Here's how the part is built. I have some questions about the finished solid (model axes, mm). A direction names the side the tool comes from. Give positions to 0.01 mm unless a question says otherwise; leave off trailing zeros. Loops run counter-clockwise (first coordinate to the right, second up) from the corner with the lowest first, then second, coordinate; pieces in that order, holes last.
Q1. I'm going to push flat-ended pins straight in: P1, Ø1.5, axis at x = -3.048, z = 0, coming from the -Y side; P2, Ø3, axis at x = -6, y = -15, coming from the -Z side; P3, Ø10, axis at x = 8, y = -18, coming from the +Z side. Where does each tip first touch, or does it pass through?
Q2. Thinking about a two-plate mould opening in Z: for faces 3 (the face through (3.25, -2.13, -0.06)), 4 (the face through (-1, -20.955, -10)), 5 (the face through (-1.83, -0.77, -0.05)), 6 (the face through (-10.418, -10.624, -3.281)), which applies, pulls with the +Z half, pulls with the -Z half, needs draft (parallel to the pull), parting line crosses it, or undercut?
Q3. Suppose I cut it at B-B (z = -3.5). List the corners of the cut face in (x, y) for me (3 decimals).
Q4. Suppose I cut it at C-C (y = -7). List the corners of the cut face in (x, z) for me, and give its area (3 significant figures).
Q5. For faces 1 (the face through (0, 0, 0)), 2 (the face through (1.885, -0.773, -0.366)), which set-ups out of +Z, -Z, +X, -X, +Y, -Y let a thin tool reach every point of the face, with its end or its side?
Q6. I need wall thicknesses on probe 1 along Y at (x, z) = (-3, 9.75) (3 decimals); probe 2 along Z at (x, y) = (0.25, -3.5); probe 3 along Z at (x, y) = (2, -8.5). Which ranges of each line are inside material? Lowest first, please.
Q7. Suppose I cut it at D-D (y = -23). List the corners of the cut face in (x, z) for me.
Q8. Suppose I cut it at A-A (x = 0). List the corners of the cut face in (y, z) for me (3 decimals), and give its area (3 significant figures).
```python
from build123d import *

# Parameters (mm, degrees)
F_2_CLEARANCE_HOLE1_D     = 2.4384
F_2_CLEARANCE_HOLE1_DEPTH = 1.524
F_2_CLEARANCE_HOLE1_TIP   = 0.732569267


with BuildPart() as part:
    # Sketch1 → Revolve1 (revolve)
    with BuildSketch(Plane.XY):
        with BuildLine():
            Line((0, 0), (-10.922, 0))
            Line((-10.922, 0), (-10.922, -20.955))
            Line((-10.922, -20.955), (-9.525, -20.955))
            ThreePointArc((-9.525, -20.955), (-6.735192091, -27.690192091), (0, -30.48))
            Line((0, -30.48), (0, 0))
        make_face()
    revolve(axis=Axis((0, 0, 0), (0, -1, 0)))

    # #2 Clearance Hole1
    with Locations(Plane(origin=(0, 0, 0), x_dir=(1, 0, 0), z_dir=(0, 1, 0))):
        with Locations((3.048, 0), (-3.048, 0)):
            Hole(F_2_CLEARANCE_HOLE1_D / 2, depth=F_2_CLEARANCE_HOLE1_DEPTH)
            with Locations((0, 0, -(F_2_CLEARANCE_HOLE1_DEPTH + F_2_CLEARANCE_HOLE1_TIP / 2))):  # 118° drill point
                Cone(0, F_2_CLEARANCE_HOLE1_D / 2, F_2_CLEARANCE_HOLE1_TIP, mode=Mode.SUBTRACT)


solid = part.part
```
Solutions:
1. P1: stops at y = -30.2
1. P2: stops at z = -9.95
1. P3: stops at z = 10.5
2. face 3: undercut
2. face 4: needs draft
2. face 5: undercut
2. face 6: parting line crosses it
3. outline: (-10.346, -20.955) - (-8.859, -20.955) arc R8.859 ccw to (8.859, -20.955) - (10.346, -20.955) - (10.346, 0) - (-10.346, 0) - close
4. outline: circle Ø21.84 at (0, 0)
4. area: 375 mm2
5. face 1: +Z, -Z, +X, -X, +Y
5. face 2: +Y
6. probe 1: y = -20.955 to 0
6. probe 2: z = -10.92 to 10.92
6. probe 3: z = -10.74 to 10.74
7. outline: circle Ø18.61 at (0, 0)
8. outline: (-20.955, -10.922) - (0, -10.922) - (0, 10.922) - (-20.955, 10.922) - (-20.955, 9.525) arc R9.525 ccw to (-20.955, -9.525) - close
8. area: 600 mm2
